CAD build for the part. Positions are in the model's coordinates, mm. A direction names the side the tool comes from. Give positions to 0.01 mm unless a question says otherwise; leave off trailing zeros. Loops run counter-clockwise (first coordinate to the right, second up) from the corner with the lowest first, then second, coordinate; pieces in that order, holes last. Notation, with made-up numbers: (-37.5, 8) - (-17.5, 8) arc R9 cw to (-17.5, 17) - close; hole circle Ø10 at (-35, 34). An arc over 180 degrees is marked (long way). Return JSON: item names as keys, results as strings.
from build123d import *

# Parameters (mm, degrees)
SKETCH_2_R          = 2.5
CUT_EXTRUDE_1_DEPTH = 22


with BuildPart() as part:
    # Эскиз1 → Повернуть1 (revolve)
    with BuildSketch(Plane.XY, mode=Mode.PRIVATE) as revolve_1_sk:
        Polygon((24, 14.784875022), (35, 14.784875022), (35, -0.215124978), (27.5, -0.215124978), (27.5, 12.784875022), (24, 12.784875022), align=None)
    revolve(revolve_1_sk.sketch.rotate(Axis((0, 60.609800664, 0), (0, -1, 0)), 90), axis=Axis((0, 60.609800664, 0), (0, -1, 0)))

    # Эскиз2 → Вырез-Вытянуть1 (cut)
    with BuildSketch(Plane.XZ.offset(0.215124978)):
        with Locations(Location((0, 31.5, 0), (0, 0, 270))):
            Circle(SKETCH_2_R)
        with Locations(Location((0, -31.5, 0), (0, 0, 270))):
            Circle(SKETCH_2_R)
        with Locations(Location((31.5, 0, 0), (0, 0, 270))):
            Circle(SKETCH_2_R)
        with Locations(Location((-31.5, 0, 0), (0, 0, 270))):
            Circle(SKETCH_2_R)
    extrude(amount=-CUT_EXTRUDE_1_DEPTH, mode=Mode.SUBTRACT)


solid = part.part
1. Cut at A-A, the plane z = 0. Write the cut outline in (x, y), plus the area to 3 significant figures.
Values follow:
{"outline": "(-35, -0.22) - (-34, -0.22) - (-34, 14.78) - (-35, 14.78) - close; (-29, -0.22) - (-27.5, -0.22) - (-27.5, 12.78) - (-24, 12.78) - (-24, 14.78) - (-29, 14.78) - close; (24, 12.78) - (27.5, 12.78) - (27.5, -0.22) - (29, -0.22) - (29, 14.78) - (24, 14.78) - close; (34, -0.22) - (35, -0.22) - (35, 14.78) - (34, 14.78) - close", "area": "89.0 mm²"}
2. Which spindle directions (+Z, -Z, +X, -X, +Y, -Y) get a long thin tool onto all of the face, cutting with end or side? Do faces 1 (the face through (-29, 7, 0)), 2 (the face through (24.397, 6.376, 12.69)). Say none if no direction does.
Values follow:
{"face 1": "+Y, -Y", "face 2": "-Y"}
3. Drill centre lines: probe 1 along X at (y, z) = (9.25, 0); probe 2 along Y at (x, z) = (26.5, -3); probe 3 along X at (y, z) = (11.75, -18). Where is each one in solid material? Low to high.
Values follow:
{"probe 1": "x = -35 to -34, -29 to -27.5, 27.5 to 29, 34 to 35", "probe 2": "y = 12.78 to 14.78", "probe 3": "x = -30.02 to -20.79, 20.79 to 30.02"}
4. Drop flat-ended pins along their axis: P1, Ø6, axis at y = 9.5, z = -3, coming from the +X side; P2, Ø6, axis at y = 8, z = 15, coming from the -X side; P3, Ø8, axis at x = -21, y = 3.5, coming from the +Z side. Give the stop position or say it passes through.
Values follow:
{"P1": "stops at x = 35", "P2": "stops at x = -32.88", "P3": "stops at z = 30.59"}
5. Cut at B-B, the plane x = -18.5. Write the cut outline in (y, z).
Values follow:
{"outline": "(-0.22, -29.71) - (14.78, -29.71) - (14.78, -15.29) - (12.78, -15.29) - (12.78, -20.35) - (-0.22, -20.35) - close; (-0.22, 20.35) - (12.78, 20.35) - (12.78, 15.29) - (14.78, 15.29) - (14.78, 29.71) - (-0.22, 29.71) - close"}
6. Cut at C-C, the plane z = 31.5. Write the cut outline in (x, y), plus the area to 3 significant figures.
Values follow:
{"outline": "(-15.26, -0.22) - (-2.5, -0.22) - (-2.5, 14.78) - (-15.26, 14.78) - close; (2.5, -0.22) - (15.26, -0.22) - (15.26, 14.78) - (2.5, 14.78) - close", "area": "383 mm²"}
7. Cut at D-D, the plane y = 9. Write the cut outline in (x, z).
Values follow:
{"outline": "circle Ø70 at (0, 0); hole circle Ø5 at (-31.5, 0); hole circle Ø55 at (0, 0); hole circle Ø5 at (0, -31.5); hole circle Ø5 at (0, 31.5); hole circle Ø5 at (31.5, 0)"}
8. Pull direction X, two halves, no side cores. Call faces 3 (the face through (-23, 12.785, -8)), 4 (the face through (34.168, 7.18, -7.587)), 5 (the face through (23, 14.785, 8)): +X half, -X half, draft (parallel to the pull), parting line (faces both ways), or undercut.
Values follow:
{"face 3": "undercut", "face 4": "parting line", "face 5": "draft"}
